from build123d import *

# Parameters (mm, degrees)
F0_R          = 3.1
F1_DEPTH      = 7
F2_DEPTH      = 15
F4_DEPTH      = 2
F4_DEPTH_BACK = 6
F5_R          = 2.1
F6_DEPTH      = 25
F8_DEPTH      = 30
F9_DEPTH      = 25
F9_DEPTH_BACK = 7
F10_R         = 3.1
F11_DEPTH     = 25
F12_R         = 5
F12_R_2       = 3.1
F13_DEPTH     = 7
F14_SIZE      = 1.99999
F15_W         = 3.459926136
F15_H         = 15.633740799
F16_DEPTH     = 25
F18_DEPTH     = 25


# Not quite as in the source:
# - a fillet or chamfer is up to 0.001 mm smaller than in the source, because OpenCascade refuses the exact size


with BuildPart() as f1:
    # F0 (on Top) → F1 (new body)
    with BuildSketch(Plane.XY):
        with BuildLine():
            ThreePointArc((-5, -21.6602540378), (-1.5866973333, -20.3139323085), (-0.0115560862, -17))
            Line((-0.0115560862, -17), (-5, -17))
            Line((-5, -17), (-5, -8.6602540378))
            ThreePointArc((-5, -8.6602540378), (-9.6592582629, 2.588190451), (0, 10))
            Line((0, 10), (0, 16.6602540378))
            ThreePointArc((0, 16.6602540378), (-1.4644660941, 20.1957879438), (-5, 21.6602540378))
            Line((-5, 21.6602540378), (-49, 21.6602540378))
            Line((-49, 21.6602540378), (-49, 0))
            Line((-49, 0), (-49, -21.6602540378))
            Line((-49, -21.6602540378), (-5, -21.6602540378))
        make_face()
        with Locations((-34, -12)):
            Circle(F0_R, mode=Mode.SUBTRACT)
        with Locations((-34, 12)):
            Circle(F0_R, mode=Mode.SUBTRACT)
    extrude(amount=F1_DEPTH)

    # F0 (on Top) → F2 (join)
    with BuildSketch(Plane.XY):
        with BuildLine():
            ThreePointArc((0, -5), (-0.50254481, 4.974680765), (1, -4.8989794856))
            Line((1, -4.8989794856), (1, -9.9498743711))
            Line((1, -9.9498743711), (1, -17))
            Line((1, -17), (6, -17))
            Line((6, -17), (6, -8))
            ThreePointArc((6, -8), (9.4868329805, 3.1622776602), (0, 10))
            ThreePointArc((0, 10), (-9.6592582629, 2.588190451), (-5, -8.6602540378))
            Line((-5, -8.6602540378), (-5, -17))
            Line((-5, -17), (-0.0115560862, -17))
            ThreePointArc((-0.0115560862, -17), (-0.0028898567, -16.8302252574), (0, -16.6602540378))
            Line((0, -16.6602540378), (0, -10))
            Line((0, -10), (0, -5))
        make_face()
    extrude(amount=F2_DEPTH)

    # F3 (on face) → F4 (cut, two sides)
    with BuildSketch(Plane(origin=(-5, 0, 0), x_dir=(0, -1, 0), z_dir=(-1, 0, 0))) as f4_sk:
        Polygon((16.3801270189, 4.9504065444), (16.3801270189, 9.0495934556), (12.8301270189, 11.0991869112), (9.2801270189, 9.0495934556), (9.2801270189, 4.9504065444), (12.8301270189, 2.9008130888), align=None)
    extrude(amount=-F4_DEPTH, mode=Mode.SUBTRACT)
    extrude(f4_sk.sketch, amount=F4_DEPTH_BACK, mode=Mode.SUBTRACT)

    # F5 (on face) → F6 (cut)
    with BuildSketch(Plane(origin=(-5, 0, 0), x_dir=(0, -1, 0), z_dir=(-1, 0, 0))):
        with Locations((12.8301270189, 7)):
            Circle(F5_R)
    extrude(amount=-F6_DEPTH, mode=Mode.SUBTRACT)

    # F7 (on face) → F8 (join)
    with BuildSketch(Plane.XY.offset(7)):
        Polygon((-19, 32.5), (-19, 21.6602540378), (-19, -21.6602540378), (-19, -32.5), (-14, -32.5), (-14, -21.6602540378), (-14, 21.6602540378), (-14, 32.5), align=None)
    extrude(amount=F8_DEPTH)

    # F7 (on face) → F9 (join, two sides)
    with BuildSketch(Plane.XY.offset(7)) as f9_sk:
        Polygon((-19, 32.5), (-19, 21.6602540378), (-19, -21.6602540378), (-19, -32.5), (-14, -32.5), (-14, -21.6602540378), (-14, 21.6602540378), (-14, 32.5), align=None)
    extrude(amount=F9_DEPTH)
    extrude(f9_sk.sketch, amount=-F9_DEPTH_BACK)

    # F10 (on face) → F11 (cut)
    with BuildSketch(Plane(origin=(-19, 0, 0), x_dir=(0, -1, 0), z_dir=(-1, 0, 0))):
        with Locations((-25, 22)):
            Circle(F10_R)
        with Locations((25, 22)):
            Circle(F10_R)
    extrude(amount=-F11_DEPTH, mode=Mode.SUBTRACT)

    # F12 (on face) → F13 (join)
    with BuildSketch(Plane(origin=(-19, 0, 0), x_dir=(0, -1, 0), z_dir=(-1, 0, 0))):
        with Locations((25, 22)):
            Circle(F12_R)
        with Locations((25, 22)):
            Circle(F12_R_2, mode=Mode.SUBTRACT)
        with Locations((-25, 22)):
            Circle(F12_R)
        with Locations((-25, 22)):
            Circle(F12_R_2, mode=Mode.SUBTRACT)
    extrude(amount=-F13_DEPTH)

    # F14 (size 2 in the source; OpenCascade refuses exactly that, so slightly less here)
    f14_edges = [f1.edges().sort_by_distance(p)[0] for p in [
        (-14, 30, 22),
        (-14, -20, 22),
    ]]
    chamfer(f14_edges, length=F14_SIZE)

    # F15 (on face) → F16 (cut)
    with BuildSketch(Plane.YZ.offset(-14)):
        with Locations((18.870036932, 22.279205732)):
            Rectangle(F15_W, F15_H)
        with Locations((-18.870036932, 22.279205732)):
            Rectangle(F15_W, F15_H)
    extrude(amount=F16_DEPTH, mode=Mode.SUBTRACT)

    # F17 (on face) → F18 (cut)
    with BuildSketch(Plane.YZ.offset(-14)):
        with BuildLine():
            Line((21.6602540378, 43.2897545397), (21.6602540378, 32.6861559824))
            ThreePointArc((21.6602540378, 32.6861559824), (27.3948854866, 32.9367434036), (32.5, 30.3125106178))
            Line((32.5, 30.3125106178), (32.5, 43.2897545397))
            Line((32.5, 43.2897545397), (21.6602540378, 43.2897545397))
        make_face()
        with BuildLine():
            ThreePointArc((-32.5, 30.3125106178), (-27.3948854866, 32.9367434036), (-21.6602540378, 32.6861559824))
            Line((-21.6602540378, 32.6861559824), (-21.6602540378, 43.2897545397))
            Line((-21.6602540378, 43.2897545397), (-32.5, 43.2897545397))
            Line((-32.5, 43.2897545397), (-32.5, 30.3125106178))
        make_face()
    extrude(amount=-F18_DEPTH, mode=Mode.SUBTRACT)


solid = f1.part
Work out the finished part from the listing and answer in its coordinate system (mm). A direction names the side the tool comes from. Give positions to 0.01 mm unless a question says otherwise; leave off trailing zeros. Loops run counter-clockwise (first coordinate to the right, second up) from the corner with the lowest first, then second, coordinate; pieces in that order, holes last. Notation, with made-up numbers: (42, 51) - (52, 51) arc R22 cw to (52, 57) - close; hole circle Ø9 at (26, 70.5). An arc over 180 degrees is marked (long way). Answer in a Markdown table with one row per item.
(1) Flat-ended cylindrical pins translate along their axes: pin 1 Ø12 at (x, z) = (-29, 21.5) entering from +Y; pin 2 Ø4 at (x, y) = (-8.5, 8) entering from +Z; pin 3 Ø11 at (y, z) = (15, 22.5) entering from +X; pin 4 Ø4.5 at (x, z) = (-8, 7.5) entering from -Y. Find the tip coordinate at first contact, or state that the pin passes through.
Results list:
| item | result |
|---|---|
| pin 1 | passes through |
| pin 2 | stops at z = 15 |
| pin 3 | stops at x = -14 |
| pin 4 | stops at y = -21.66 |
(2) For a pull along Z with two mould halves and no side action, classify faces 4 (the face through (-17, 0, 37)), 5 (the face through (-1.521, -12.557, 9.082)), 6 (the face through (-49, 0, 3)) as pulls with the +Z half, pulls with the -Z half, needs draft (parallel to the pull), parting line crosses it, or undercut.
Results list:
| item | result |
|---|---|
| face 4 | pulls with the +Z half |
| face 5 | undercut |
| face 6 | needs draft |
(3) Consider L1, parallel to Z at x = -17.5, y = 25; L2, parallel to X at y = 3, z = 9; L3, parallel to Z at x = -2, y = 7.5. Determine where each line is inside the solid, lowest interval first. Write a range as [from, to].
Results list:
| item | result |
|---|---|
| L1 | z = [0, 18.9], [25.1, 33.2] |
| L2 | x = [-19, -14], [-9.54, -4], [4, 9.54] |
| L3 | z = [0, 15] |
(4) Section B-B (x = -34) is taken. Give the vertices of the cut face in (y, z), and give its area (3 significant figures).
Results list:
| item | result |
|---|---|
| outline | (-21.66, 0) - (-15.1, 0) - (-15.1, 7) - (-21.66, 7) - close; (-8.9, 0) - (8.9, 0) - (8.9, 7) - (-8.9, 7) - close; (15.1, 0) - (21.66, 0) - (21.66, 7) - (15.1, 7) - close |
| area | 216 mm² |
(5) Section D-D (x = -9) is taken. Give the vertices of the cut face in (y, z), and give its area (3 significant figures).
Results list:
| item | result |
|---|---|
| outline | (-21.66, 0) - (21.66, 0) - (21.66, 7) - (4.36, 7) - (4.36, 15) - (-4.36, 15) - (-4.36, 7) - (-9.28, 7) - (-9.28, 4.95) - (-12.83, 2.9) - (-16.38, 4.95) - (-16.38, 7) - (-21.66, 7) - close |
| area | 351 mm² |
(6) Section A-A (y = 12) is taken. Give the vertices of the cut face in (x, z).
Results list:
| item | result |
|---|---|
| outline | (-49, 0) - (-37.1, 0) - (-37.1, 7) - (-49, 7) - close; (-30.9, 0) - (0, 0) - (0, 7) - (-14, 7) - (-14, 37) - (-19, 37) - (-19, 7) - (-30.9, 7) - close |
(7) A tool of negligible diameter and unlimited length cuts with its end or side. For faces 1 (the face through (-12, 27.5, 19.8)), 2 (the face through (-4.01, -14.63, 10.06)), 3 (the face through (3.465, -12.557, 9.082)), from which of +Z, -Z, +X, -X, +Y, -Y can it reach the whole face along a straight path? Write none if from no direction.
Results list:
| item | result |
|---|---|
| face 1 | +Z, +X, +Y, -Y |
| face 2 | none |
| face 3 | +X |
